The model under review builds one solid part; all positions refer to its coordinate system, in mm. A direction names the side the tool comes from. Round coordinates to 2 decimals unless told otherwise and drop trailing zeros. Write each loop counter-clockwise with the first axis right and the second up, starting at its lowest first coordinate (ties: lowest second). Pieces come first, ordered by that corner, then holes.
Item 1: Draft analysis for pull direction Y (two halves, no side actions). For faces 4 (the face through (120.672, 35.07, 34.662)), 5 (the face through (75, 114, 33)), 6 (the face through (37, 85, 35)), state which applies: +Y half, -Y half, draft (parallel to the pull), parting line (faces both ways), or undercut.
Item 2: Add section B-B (y = 105.5). State how many separate pieces and enclosed holes the cut face has, plus the area to 3 significant figures.
Item 3: To check wall thickness, follow L1, parallel to X at y = 98, z = 34.5; L2, parallel to Y at x = 98, z = 47.5; L3, parallel to Y at x = 127.5, z = 27. State the ranges of each line that lie inside material, in increasing order.
Item 4: Add section D-D (x = 132). Give the boundary of the cut face in (y, z).
Item 5: Machinability: for faces 1 (the face through (143, 60, 35)), 2 (the face through (20, 97, 45)), 3 (the face through (20, 100.155, 33)), which of the approach directions +Z, -Z, +X, -X, +Y, -Y give a long, thin tool a straight path to every point of the face, cutting with its end or side? Answer none if there is none.
Item 6: Add section C-C (y = 64). Give the boundary of the cut face in (x, z), plus the area to 3 significant figures.
Item 7: Clearance check with flat-ended pins moving along their axes: pin 1 Ø10 at (x, y) = (90, 31) entering from -Z; pin 2 Ø3 at (x, y) = (8, 51.5) entering from +Z; pin 3 Ø8 at (y, z) = (55, 58.5) entering from +X. State where each tip first meets the part, or that it passes through.
Item 8: Add section A-A (x = 149). Give the boundary of the cut face in (y, z), plus the area to 3 significant figures.
```python
from build123d import *

# Parameters (mm, degrees)
SKETCH1_W                = 150
SKETCH1_H                = 120
BOSS_EXTRUDE2_DEPTH      = 70
BOSS_EXTRUDE5_DEPTH      = 3
BOSS_EXTRUDE5_DEPTH_BACK = 7
SKETCH4_W                = 168
SKETCH4_H                = 150
SKETCH6_R                = 3.1
CUT_EXTRUDE1_DEPTH       = 20
FILLET2_R                = 5
SKETCH2_R                = 20.1
CUT_EXTRUDE2_DEPTH       = 9.5
SKETCH9_R                = 5
CUT_EXTRUDE5_DEPTH       = 20
SKETCH15_W               = 167.384372829
SKETCH15_H               = 135.598337876
CUT_EXTRUDE12_DEPTH      = 10
SKETCH16_W               = 75
SKETCH16_H               = 88
CUT_EXTRUDE13_DEPTH      = 50
BOSS_EXTRUDE6_START      = 55
SKETCH18_W               = 75
SKETCH18_H               = 50
BOSS_EXTRUDE6_DEPTH      = 10
CUT_EXTRUDE14_START      = -25
SKETCH17_R               = 5.1
CUT_EXTRUDE14_DEPTH      = 17
CUT_EXTRUDE15_START      = -25
SKETCH17_3_R             = 2.6
CUT_EXTRUDE15_DEPTH      = 90
SKETCH19_W               = 50
SKETCH19_H               = 35
CUT_EXTRUDE19_DEPTH      = 56.62
CUT_EXTRUDE20_DEPTH      = 46
CUT_EXTRUDE21_START      = -60
SKETCH21_R               = 2
CUT_EXTRUDE21_DEPTH      = 25
SKETCH9_4_R              = 5
CUT_EXTRUDE24_DEPTH      = 150
CUT_EXTRUDE25_START      = -10
SKETCH22_W               = 10
SKETCH22_H               = 30
CUT_EXTRUDE25_DEPTH      = 29
SKETCH23_R               = 2.1
CUT_EXTRUDE26_DEPTH      = 243.458243828
CUT_EXTRUDE27_START      = -10
SKETCH23_3_R             = 4
CUT_EXTRUDE27_DEPTH      = 5
SKETCH24_R               = 1.5
CUT_EXTRUDE28_DEPTH      = 30
SKETCH25_W               = 10
SKETCH25_H               = 30
CUT_EXTRUDE29_DEPTH      = 40
CUT_EXTRUDE30_DEPTH      = 196
CUT_EXTRUDE32_DEPTH      = 196
CUT_EXTRUDE33_START      = -3
SKETCH30_W               = 8.52
SKETCH30_H               = 40
CUT_EXTRUDE33_DEPTH      = 37
FILLET3_R                = 5
CUT_EXTRUDE34_START      = -3
SKETCH31_W               = 5.550839789
SKETCH31_H               = 10.134989035
SKETCH31_W_2             = 14.692790928
SKETCH31_H_2             = 12.94032263
CUT_EXTRUDE34_DEPTH      = 49
SKETCH32_W               = 8.5
SKETCH32_H               = 8.5
CUT_EXTRUDE37_DEPTH      = 5


with BuildPart() as part:
    # Sketch1 → Boss-Extrude2 (new body)
    with BuildSketch(Plane.XY):
        with Locations((75, 60)):
            Rectangle(SKETCH1_W, SKETCH1_H)
    extrude(amount=BOSS_EXTRUDE2_DEPTH)

    # Sketch4 → Boss-Extrude5 (add, two sides: drawn at the far end of the back side and taken through both)
    with BuildSketch(Plane.XZ.offset(-BOSS_EXTRUDE5_DEPTH_BACK)):
        with Locations((75, 69)):
            Rectangle(SKETCH4_W, SKETCH4_H)
    extrude(amount=BOSS_EXTRUDE5_DEPTH + BOSS_EXTRUDE5_DEPTH_BACK)

    # Sketch6 → Cut-Extrude1 (cut)
    with BuildSketch(Plane.XZ.offset(3)):
        with Locations((1, 134)):
            Circle(SKETCH6_R)
        with Locations((149, 134)):
            Circle(SKETCH6_R)
        with Locations((149, 4)):
            Circle(SKETCH6_R)
        with Locations((1, 4)):
            Circle(SKETCH6_R)
    extrude(amount=-CUT_EXTRUDE1_DEPTH, mode=Mode.SUBTRACT)

    # Fillet2
    fillet2_edges = [part.edges().sort_by_distance(p)[0] for p in [
        (-9, 2, -6),
        (-9, 7, 69),
        (-9, 2, 144),
        (75, 7, 144),
        (159, 2, 144),
        (159, 7, 69),
        (159, 2, -6),
        (75, 7, -6),
    ]]
    fillet(fillet2_edges, radius=FILLET2_R)

    # Sketch2 → Cut-Extrude2 (cut)
    with BuildSketch(Plane(origin=(0, 120, 0), x_dir=(1, 0, 0), z_dir=(0, 1, 0))):
        with Locations(Location((105, -35, 0), (0, 0, 270))):
            Circle(SKETCH2_R)
    extrude(amount=-CUT_EXTRUDE2_DEPTH, mode=Mode.SUBTRACT)

    # Sketch9 → Cut-Extrude5 (cut)
    with BuildSketch(Plane(origin=(0, 110.5, 0), x_dir=(1, 0, 0), z_dir=(0, 1, 0))):
        with Locations(Location((105, -35, 0), (0, 0, 270))):
            Circle(SKETCH9_R)
    extrude(amount=-CUT_EXTRUDE5_DEPTH, mode=Mode.SUBTRACT)

    # Sketch15 → Cut-Extrude12 (cut)
    with BuildSketch(Plane.XY.offset(70)):
        with Locations((79.692186415, 74.799168938)):
            Rectangle(SKETCH15_W, SKETCH15_H)
    extrude(amount=-CUT_EXTRUDE12_DEPTH, mode=Mode.SUBTRACT)

    # Sketch16 → Cut-Extrude13 (cut)
    with BuildSketch(Plane.XY.offset(60)):
        with Locations((102.5, 51)):
            Rectangle(SKETCH16_W, SKETCH16_H)
    extrude(amount=-CUT_EXTRUDE13_DEPTH, mode=Mode.SUBTRACT)

    # Sketch18 → Boss-Extrude6 (add)
    with BuildSketch(Plane.XZ.offset(-95).offset(BOSS_EXTRUDE6_START)):
        with Locations((102.5, 35)):
            Rectangle(SKETCH18_W, SKETCH18_H)
    extrude(amount=BOSS_EXTRUDE6_DEPTH)

    # Sketch17 → Cut-Extrude14 (cut)
    with BuildSketch(Plane.XZ.offset(-95).offset(CUT_EXTRUDE14_START)):
        with Locations(Location((123.25, 35, 0), (0, 0, 76.030533487))):
            Circle(SKETCH17_R)
        with Locations(Location((86.75, 35, 0), (0, 0, 103.969466513))):
            Circle(SKETCH17_R)
    extrude(amount=CUT_EXTRUDE14_DEPTH, mode=Mode.SUBTRACT)

    # Sketch17<3> → Cut-Extrude15 (cut)
    with BuildSketch(Plane.XZ.offset(-95).offset(CUT_EXTRUDE15_START)):
        with Locations(Location((123.25, 35, 0), (0, 0, 90))):
            Circle(SKETCH17_3_R)
        with Locations(Location((86.75, 35, 0), (0, 0, 90))):
            Circle(SKETCH17_3_R)
    extrude(amount=CUT_EXTRUDE15_DEPTH, mode=Mode.SUBTRACT)

    # Sketch19 → Cut-Extrude19 (cut)
    with BuildSketch(Plane(origin=(65, 0, 0), x_dir=(0, 0, -1), z_dir=(1, 0, 0))):
        with Locations((-35, 67.5)):
            Rectangle(SKETCH19_W, SKETCH19_H)
    extrude(amount=-CUT_EXTRUDE19_DEPTH, mode=Mode.SUBTRACT)

    # Sketch20 → Cut-Extrude20 (cut)
    with BuildSketch(Plane.XY.offset(60)):
        Polygon((8.38, 8), (50.48, 8), (50.48, 58), (33.43, 58), (33.43, 83), (25.43, 83), (25.43, 58), (8.38, 58), align=None)
    extrude(amount=-CUT_EXTRUDE20_DEPTH, mode=Mode.SUBTRACT)

    # Sketch21 → Cut-Extrude21 (cut)
    with BuildSketch(Plane(origin=(0, 0, 0), x_dir=(-1, 0, 0), z_dir=(0, 0, -1)).offset(CUT_EXTRUDE21_START)):
        with Locations((-20, 95)):
            Circle(SKETCH21_R)
        with Locations((-105, 35)):
            Circle(SKETCH21_R)
        with Locations((-55, 95)):
            Circle(SKETCH21_R)
    extrude(amount=CUT_EXTRUDE21_DEPTH, mode=Mode.SUBTRACT)

    # Sketch9<4> → Cut-Extrude24 (cut)
    with BuildSketch(Plane(origin=(0, 110.5, 0), x_dir=(1, 0, 0), z_dir=(0, 1, 0))):
        with Locations(Location((105, -35, 0), (0, 0, 270))):
            Circle(SKETCH9_4_R)
    extrude(amount=-CUT_EXTRUDE24_DEPTH, mode=Mode.SUBTRACT)

    # Sketch22 → Cut-Extrude25 (cut)
    with BuildSketch(Plane(origin=(0, 40, 0), x_dir=(1, 0, 0), z_dir=(0, 1, 0)).offset(CUT_EXTRUDE25_START)):
        with Locations((70, -35)):
            Rectangle(SKETCH22_W, SKETCH22_H)
    extrude(amount=CUT_EXTRUDE25_DEPTH, mode=Mode.SUBTRACT)

    # Sketch23 → Cut-Extrude26 (cut, through all)
    with BuildSketch(Plane(origin=(0, 7, 0), x_dir=(1, 0, 0), z_dir=(0, 1, 0))):
        with Locations(Location((24.822097221, -72.904396363, 0), (0, 0, 180))):
            Circle(SKETCH23_R)
        with Locations(Location((97.135530056, -72.904396363, 0), (0, 0, 180))):
            Circle(SKETCH23_R)
        with Locations(Location((97.135530056, -129.904396363, 0), (0, 0, 180))):
            Circle(SKETCH23_R)
    extrude(amount=-CUT_EXTRUDE26_DEPTH, mode=Mode.SUBTRACT)

    # Sketch23<3> → Cut-Extrude27 (cut)
    with BuildSketch(Plane(origin=(0, 7, 0), x_dir=(1, 0, 0), z_dir=(0, 1, 0)).offset(CUT_EXTRUDE27_START)):
        with Locations(Location((24.822097221, -72.904396363, 0), (0, 0, 180))):
            Circle(SKETCH23_3_R)
        with Locations(Location((97.135530056, -72.904396363, 0), (0, 0, 180))):
            Circle(SKETCH23_3_R)
        with Locations(Location((97.135530056, -129.904396363, 0), (0, 0, 180))):
            Circle(SKETCH23_3_R)
    extrude(amount=CUT_EXTRUDE27_DEPTH, mode=Mode.SUBTRACT)

    # Sketch24 → Cut-Extrude28 (cut)
    with BuildSketch(Plane(origin=(0, 120, 0), x_dir=(1, 0, 0), z_dir=(0, 1, 0))):
        with Locations(Location((61.5, -36.5, 0), (0, 0, 270))):
            Circle(SKETCH24_R)
        with Locations(Location((61.5, -56.5, 0), (0, 0, 270))):
            Circle(SKETCH24_R)
    extrude(amount=-CUT_EXTRUDE28_DEPTH, mode=Mode.SUBTRACT)

    # Sketch25 → Cut-Extrude29 (cut)
    with BuildSketch(Plane(origin=(0, 120, 0), x_dir=(1, 0, 0), z_dir=(0, 1, 0))):
        with Locations((44.48, -35)):
            Rectangle(SKETCH25_W, SKETCH25_H)
    extrude(amount=-CUT_EXTRUDE29_DEPTH, mode=Mode.SUBTRACT)

    # Sketch27 → Cut-Extrude30 (cut)
    with BuildSketch(Plane.XY.offset(60)):
        Polygon((143, 114), (5.38, 114), (5.38, 7), (-15.039720256, 7), (-15.039720256, 109), (-15.039720256, 126.65195416), (160.466879019, 126.65195416), (160.466879019, 109), (160.466879019, 7), (143, 7), align=None)
    extrude(amount=-CUT_EXTRUDE30_DEPTH, mode=Mode.SUBTRACT)

    # Sketch29 → Cut-Extrude32 (cut)
    with BuildSketch(Plane.ZY.offset(-5.38)):
        Polygon((-8.937501462, 135.391592563), (5, 135.391592563), (5, 7), (-13.483359674, 7), align=None)
    extrude(amount=-CUT_EXTRUDE32_DEPTH, mode=Mode.SUBTRACT)

    # Sketch30 → Cut-Extrude33 (cut)
    with BuildSketch(Plane(origin=(0, 50, 0), x_dir=(1, 0, 0), z_dir=(0, 1, 0)).offset(CUT_EXTRUDE33_START)):
        with Locations((57.74, -37)):
            Rectangle(SKETCH30_W, SKETCH30_H)
    extrude(amount=-CUT_EXTRUDE33_DEPTH, mode=Mode.SUBTRACT)

    # Fillet3
    fillet3_edges = [part.edges().sort_by_distance(p)[0] for p in [
        (143, 60.5, 5),
        (5.38, 60.5, 5),
    ]]
    fillet(fillet3_edges, radius=FILLET3_R)

    # Sketch31 → Cut-Extrude34 (cut)
    with BuildSketch(Plane.XY.offset(60).offset(CUT_EXTRUDE34_START)):
        Polygon((37.902832863, 110.401622614), (25.54931853, 110.401622614), (13.735368308, 110.401622614), (13.735368308, 100.155334019), (25.54931853, 100.155334019), (25.54931853, 87.423968607), (37.902832863, 87.423968607), align=None)
        with Locations((55.5860526, 105.941968642)):
            Rectangle(SKETCH31_W, SKETCH31_H)
        with Locations((73.077247019, 104.554579716)):
            Rectangle(SKETCH31_W_2, SKETCH31_H_2)
    extrude(amount=-CUT_EXTRUDE34_DEPTH, mode=Mode.SUBTRACT)

    # Sketch32 → Cut-Extrude37 (cut)
    with BuildSketch(Plane.XY.offset(60)):
        with Locations((20, 95)):
            Rectangle(SKETCH32_W, SKETCH32_H)
        with Locations((55, 95)):
            Rectangle(SKETCH32_W, SKETCH32_H)
        with Locations((105, 35)):
            Rectangle(SKETCH32_W, SKETCH32_H)
    extrude(amount=-CUT_EXTRUDE37_DEPTH, mode=Mode.SUBTRACT)


solid = part.part
```
Numbers:
1. face 4: draft
1. face 5: +Y half
1. face 6: undercut
2. separate pieces: 1
2. enclosed holes: 9
2. area: 4,830 mm2
3. L1: x = 5.38 to 25.55, 37.9 to 39.48, 49.48 to 84.2, 89.3 to 100.03, 109.97 to 120.7, 125.8 to 143
3. L2: y = -3 to 7, 30 to 40, 95 to 110.5
3. L3: y = -3 to 7, 30 to 40, 95 to 114
4. outline: (-3, -6) - (2, -6) arc R5 ccw to (7, -1) - (7, 5) - (114, 5) - (114, 60) - (95, 60) - (95, 10) - (40, 10) - (40, 60) - (30, 60) - (30, 10) - (7, 10) - (7, 139) arc R5 ccw to (2, 144) - (-3, 144) - close
5. face 1: +Z, -Z, +X, +Y
5. face 2: +Z
5. face 3: none
6. outline: (5.38, 10) arc R5 ccw to (10.38, 5) - (138, 5) arc R5 ccw to (143, 10) - (143, 60) - (140, 60) - (140, 10) - (8.38, 10) - (8.38, 60) - (5.38, 60) - close
6. area: 977 mm2
7. pin 1: stops at z = 5
7. pin 2: stops at z = 60
7. pin 3: stops at x = 143
8. outline: (-3, -6) - (2, -6) arc R5 ccw to (7, -1) - (7, 0.9) - (-3, 0.9) - close; (-3, 7.1) - (7, 7.1) - (7, 130.9) - (-3, 130.9) - close; (-3, 137.1) - (7, 137.1) - (7, 139) arc R5 ccw to (2, 144) - (-3, 144) - close
8. area: 1,370 mm2
